```python
from build123d import *

# Parameters (mm, degrees)
SKETCH1_R           = 13
SKETCH1_R_2         = 1.375
SKETCH1_R_3         = 5
BOSS_EXTRUDE1_DEPTH = 3
SKETCH2_R           = 7.5
SKETCH2_R_2         = 5
BOSS_EXTRUDE2_DEPTH = 10
SKETCH3_R           = 5.25
CUT_EXTRUDE1_DEPTH  = 18
CUT_EXTRUDE2_DEPTH  = 4
CUT_EXTRUDE3_START  = -10
SKETCH5_R           = 7.5
SKETCH5_R_2         = 7.45
CUT_EXTRUDE3_DEPTH  = 10


with BuildPart() as part:
    # Sketch1 → Boss-Extrude1 (new body)
    with BuildSketch(Plane(origin=(0, 0, 0), x_dir=(1, 0, 0), z_dir=(0, 1, 0))):
        with Locations(Location((0, 0, 0), (0, 0, 270))):
            Circle(SKETCH1_R)
        with Locations(Location((0, 11, 0), (0, 0, 270))):
            Circle(SKETCH1_R_2, mode=Mode.SUBTRACT)
        with Locations(Location((7.778174593, 7.778174593, 0), (0, 0, 270))):
            Circle(SKETCH1_R_2, mode=Mode.SUBTRACT)
        with Locations(Location((11, 0, 0), (0, 0, 270))):
            Circle(SKETCH1_R_2, mode=Mode.SUBTRACT)
        with Locations(Location((7.778174593, -7.778174593, 0), (0, 0, 270))):
            Circle(SKETCH1_R_2, mode=Mode.SUBTRACT)
        with Locations(Location((0, -11, 0), (0, 0, 270))):
            Circle(SKETCH1_R_2, mode=Mode.SUBTRACT)
        with Locations(Location((-7.778174593, -7.778174593, 0), (0, 0, 270))):
            Circle(SKETCH1_R_2, mode=Mode.SUBTRACT)
        with Locations(Location((-11, 0, 0), (0, 0, 270))):
            Circle(SKETCH1_R_2, mode=Mode.SUBTRACT)
        with Locations(Location((-7.778174593, 7.778174593, 0), (0, 0, 270))):
            Circle(SKETCH1_R_2, mode=Mode.SUBTRACT)
        with Locations(Location((0, 0, 0), (0, 0, 270))):
            Circle(SKETCH1_R_3, mode=Mode.SUBTRACT)
    extrude(amount=BOSS_EXTRUDE1_DEPTH)

    # Sketch2 → Boss-Extrude2 (add)
    with BuildSketch(Plane(origin=(0, 3, 0), x_dir=(1, 0, 0), z_dir=(0, 1, 0))):
        with Locations(Location((0, 0, 0), (0, 0, 270))):
            Circle(SKETCH2_R)
        with Locations(Location((0, 0, 0), (0, 0, 270))):
            Circle(SKETCH2_R_2, mode=Mode.SUBTRACT)
    extrude(amount=BOSS_EXTRUDE2_DEPTH)

    # Sketch3 → Cut-Extrude1 (cut)
    with BuildSketch(Plane(origin=(0, 13, 0), x_dir=(1, 0, 0), z_dir=(0, 1, 0))):
        with Locations(Location((0, 0, 0), (0, 0, 270))):
            Circle(SKETCH3_R)
    extrude(amount=-CUT_EXTRUDE1_DEPTH, mode=Mode.SUBTRACT)

    # Sketch4 → Cut-Extrude2 (cut)
    with BuildSketch(Plane(origin=(0, 13, 0), x_dir=(1, 0, 0), z_dir=(0, 1, 0))):
        with BuildLine():
            Line((0, 5.25), (0, 7.5))
            ThreePointArc((0, 7.5), (-7.5, 0), (0, -7.5))
            Line((0, -7.5), (0, -5.25))
            ThreePointArc((0, -5.25), (-5.25, 0), (0, 5.25))
        make_face()
    extrude(amount=-CUT_EXTRUDE2_DEPTH, mode=Mode.SUBTRACT)

    # Sketch5 → Cut-Extrude3 (cut)
    with BuildSketch(Plane(origin=(0, 13, 0), x_dir=(1, 0, 0), z_dir=(0, 1, 0)).offset(CUT_EXTRUDE3_START)):
        Circle(SKETCH5_R)
        with Locations(Location((0, 0, 0), (0, 0, 270))):
            Circle(SKETCH5_R_2, mode=Mode.SUBTRACT)
    extrude(amount=CUT_EXTRUDE3_DEPTH, mode=Mode.SUBTRACT)


solid = part.part
```
Geometry: final body of the model. Coordinates: model frame, mm. A direction names the side the tool comes from. Round coordinates to 2 decimals unless told otherwise and drop trailing zeros. Order: outer loops, then holes, each group sorted by start corner. A loop starts at its lowest first (then second) coordinate and runs counter-clockwise, first axis right, second up. Notation, with made-up numbers: (-24.5, 73.25) -> (19.5, 73.25) arc R10 ccw to (19.5, 89.25) -> close; hole circle Ø7 at (-21.5, 22). An arc over 180 degrees is marked (long way). Use CSV: the item, a comma, the result in double quotes. Start each with the question number.
1) Section D-D (y = 4.25). Return the cut outline in (x, z), and give its area (3 significant figures).
2) Draft query along X for faces 1 (the face through (7.387, 6.819, -0.97)), 2 (the face through (-5.4, 9, -0.1)), 3 (the face through (-9, 1.48, 8.41)). Return one class per face: +X half, -X half, draft (parallel to the pull), parting line (faces both ways), or undercut.
3) Section B-B (x = 8.75). Return the cut outline in (y, z), and give its area (3 significant figures).
4) Set-up query: faces 4 (the face through (0, 0, 6)), 5 (the face through (-6, 3, 6)), 6 (the face through (0, 11, 6)). Return all of +Z, -Z, +X, -X, +Y, -Y with unobstructed straight access to the full face (end or side cutting, diameter ignored); none if empty.
5) Section C-C (z = 10.75). Return the cut outline in (x, y).
6) First-contact query: pin 1 Ø8 at (x, z) = (-2, 1.5) entering from +Y; pin 2 Ø6 at (x, y) = (-7, 5.5) entering from +Z; pin 3 Ø3.5 at (x, z) = (-11, 0) entering from +Y. Flat tips, straight axial feed; report the tip coordinate or a pass-through.
7) Section A-A (z = 0). Return the cut outline in (x, y) (3 decimals).
8) Material intervals for line 1 along X through (y, z) = (2, 0) (3 decimals); line 2 along X through (y, z) = (0.5, 8); line 3 along Z through (x, y) = (-8.75, 1.5), sorted ascending. Write a range as from..to.
Returned:
1,outline,"circle Ø14.9 at (0, 0); hole circle Ø10.5 at (0, 0)"
1,area,"87.8 mm²"
2,face 1,"parting line"
2,face 2,"draft"
2,face 3,"undercut"
3,outline,"(0, -9.61) -> (3, -9.61) -> (3, -8.75) -> (0, -8.75) -> close; (0, -6.81) -> (3, -6.81) -> (3, 6.81) -> (0, 6.81) -> close; (0, 8.75) -> (3, 8.75) -> (3, 9.61) -> (0, 9.61) -> close"
3,area,"46.0 mm²"
4,face 4,"+Z, -Z, +X, -X, -Y"
4,face 5,"+Y"
4,face 6,"+Z, -Z, -X, +Y"
5,outline,"(-7.31, 0) -> (-1.35, 0) -> (-1.35, 3) -> (-7.31, 3) -> close; (1.35, 0) -> (7.31, 0) -> (7.31, 3) -> (1.35, 3) -> close"
6,pin 1,"stops at y = 9"
6,pin 2,"stops at z = 11.85"
6,pin 3,"stops at y = 3"
7,outline,"(-13, 0) -> (-12.375, 0) -> (-12.375, 3) -> (-13, 3) -> close; (-9.625, 0) -> (-5.25, 0) -> (-5.25, 9) -> (-7.45, 9) -> (-7.45, 3) -> (-9.625, 3) -> close; (5.25, 0) -> (9.625, 0) -> (9.625, 3) -> (7.45, 3) -> (7.45, 13) -> (5.25, 13) -> close; (12.375, 0) -> (13, 0) -> (13, 3) -> (12.375, 3) -> close"
8,line 1,"x = -13..-12.375, -9.625..-5.25, 5.25..9.625, 12.375..13"
8,line 2,"x = -10.25..-9.14, -6.42..6.42, 9.14..10.25"
8,line 3,"z = -9.61..-8.75, -6.81..6.81, 8.75..9.61"
